```python
from build123d import *

# Parameters (mm, degrees)
RESSALTO_EXTRUS_O1_DEPTH   = 5
ESBO_O2_R                  = 1.35
ESBO_O2_R_2                = 1.373066436
ESBO_O2_R_3                = 1.330065432
ESBO_O2_R_4                = 5
CORTE_EXTRUS_O1_DEPTH      = 137.810087347
ESBO_O3_R                  = 5
CORTE_EXTRUS_O2_DEPTH      = 137.810087347
ESBO_O5_W                  = 31.24115408
ESBO_O5_H                  = 28
CORTE_EXTRUS_O3_DEPTH      = 137.810087347
ESBO_O6_W                  = 5
ESBO_O6_H                  = 28
RESSALTO_EXTRUS_O2_DEPTH   = 2.5
RESSALTO_EXTRUS_O4_DEPTH   = 5
ESBO_O8_R                  = 5
ESBO_O8_R_2                = 1.35
CORTE_EXTRUS_O4_DEPTH      = 135.937948702
ESBO_O10_W                 = 5
ESBO_O10_H                 = 2.5
CORTE_EXTRUS_O5_DEPTH      = 137.985400682
ESBO_O11_W                 = 5
ESBO_O11_H                 = 2.5
RESSALTO_EXTRUS_O5_DEPTH   = 28
ESBO_O14_W                 = 51.545841804
ESBO_O14_H                 = 28
CORTE_EXTRUS_O6_DEPTH      = 10
CORTE_EXTRUS_O7_DEPTH      = 135.822105012
CORTE_EXTRUS_O7_DEPTH_BACK = 10
ESBO_O16_R                 = 5
CORTE_EXTRUS_O8_DEPTH      = 10


with BuildPart() as part:
    # Esboço1 → Ressalto-extrusão1 (new body)
    with BuildSketch(Plane.XY):
        with BuildLine():
            Line((0, -14), (122, -14))
            ThreePointArc((122, -14), (136, 0), (122, 14))
            Line((122, 14), (0, 14))
            ThreePointArc((0, 14), (-14, 0), (0, -14))
        make_face()
    extrude(amount=RESSALTO_EXTRUS_O1_DEPTH)

    # Esboço2 → Corte-extrusão1 (cut, through all)
    with BuildSketch(Plane(origin=(0, 0, 0), x_dir=(-1, 0, 0), z_dir=(0, 0, -1))):
        with Locations((-125.327123404, 10.484762747)):
            Circle(ESBO_O2_R)
        with Locations((-116.938784683, 9.766478358)):
            Circle(ESBO_O2_R)
        with Locations((-111.515237253, 3.327123404)):
            Circle(ESBO_O2_R)
        with Locations((-112.233521642, -5.061215317)):
            Circle(ESBO_O2_R)
        with Locations((-118.672876596, -10.484762747)):
            Circle(ESBO_O2_R_2)
        with Locations((-127.061215317, -9.766478358)):
            Circle(ESBO_O2_R_3)
        with Locations((-132.484762747, -3.327123404)):
            Circle(ESBO_O2_R)
        with Locations((-131.766478358, 5.061215317)):
            Circle(ESBO_O2_R)
        with Locations((-122, 0)):
            Circle(ESBO_O2_R_4)
    extrude(amount=-CORTE_EXTRUS_O1_DEPTH, mode=Mode.SUBTRACT)

    # Esboço3 → Corte-extrusão2 (cut, through all)
    with BuildSketch(Plane(origin=(0, 0, 0), x_dir=(-1, 0, 0), z_dir=(0, 0, -1))):
        Circle(ESBO_O3_R)
    extrude(amount=-CORTE_EXTRUS_O2_DEPTH, mode=Mode.SUBTRACT)

    # Esboço5 → Corte-extrusão3 (cut, through all)
    with BuildSketch(Plane(origin=(0, 0, 0), x_dir=(-1, 0, 0), z_dir=(0, 0, -1))):
        with Locations((-121.62057704, 0)):
            Rectangle(ESBO_O5_W, ESBO_O5_H)
    extrude(amount=-CORTE_EXTRUS_O3_DEPTH, mode=Mode.SUBTRACT)

    # Esboço6 → Ressalto-extrusão2 (add)
    with BuildSketch(Plane(origin=(0, 0, 0), x_dir=(-1, 0, 0), z_dir=(0, 0, -1))):
        with Locations((-103.5, 0)):
            Rectangle(ESBO_O6_W, ESBO_O6_H)
    extrude(amount=RESSALTO_EXTRUS_O2_DEPTH)

    # Esboço7 → Ressalto-extrusão4 (add)
    with BuildSketch(Plane(origin=(0, 0, -2.5), x_dir=(-1, 0, 0), z_dir=(0, 0, -1))):
        with BuildLine():
            Line((-106, 14), (-120, 14))
            ThreePointArc((-120, 14), (-134, 0), (-120, -14))
            Line((-120, -14), (-106, -14))
            Line((-106, -14), (-106, 14))
        make_face()
    extrude(amount=-RESSALTO_EXTRUS_O4_DEPTH)

    # Esboço8 → Corte-extrusão4 (cut, through all)
    with BuildSketch(Plane(origin=(0, 0, -2.5), x_dir=(-1, 0, 0), z_dir=(0, 0, -1))):
        with Locations((-120, 0)):
            Circle(ESBO_O8_R)
        with Locations((-120, 11)):
            Circle(ESBO_O8_R_2)
        with Locations((-109, 0)):
            Circle(ESBO_O8_R_2)
        with Locations((-120, -11)):
            Circle(ESBO_O8_R_2)
        with Locations((-131, 0)):
            Circle(ESBO_O8_R_2)
        with Locations((-112.221825407, 7.778174593)):
            Circle(ESBO_O8_R_2)
        with Locations((-112.221825407, -7.778174593)):
            Circle(ESBO_O8_R_2)
        with Locations((-127.778174593, -7.778174593)):
            Circle(ESBO_O8_R_2)
        with Locations((-127.778174593, 7.778174593)):
            Circle(ESBO_O8_R_2)
    extrude(amount=-CORTE_EXTRUS_O4_DEPTH, mode=Mode.SUBTRACT)

    # Esboço10 → Corte-extrusão5 (cut, through all)
    with BuildSketch(Plane.XZ.offset(14)):
        with Locations((103.5, 3.75)):
            Rectangle(ESBO_O10_W, ESBO_O10_H)
    extrude(amount=-CORTE_EXTRUS_O5_DEPTH, mode=Mode.SUBTRACT)

    # Esboço11 → Ressalto-extrusão5 (add, through all)
    with BuildSketch(Plane.XZ.offset(14)):
        with Locations((98.5, -1.25)):
            Rectangle(ESBO_O11_W, ESBO_O11_H)
    extrude(amount=-RESSALTO_EXTRUS_O5_DEPTH)

    # Esboço14 → Corte-extrusão6 (cut)
    with BuildSketch(Plane(origin=(0, 0, 0), x_dir=(-1, 0, 0), z_dir=(0, 0, -1))):
        with Locations((-10.227079098, 0)):
            Rectangle(ESBO_O14_W, ESBO_O14_H)
    extrude(amount=-CORTE_EXTRUS_O6_DEPTH, mode=Mode.SUBTRACT)

    # Esboço15 → Corte-extrusão7 (cut, two sides: drawn at the far end of the back side and taken through both)
    with BuildSketch(Plane(origin=(0, 0, 0), x_dir=(-1, 0, 0), z_dir=(0, 0, -1)).offset(-CORTE_EXTRUS_O7_DEPTH_BACK)):
        with BuildLine():
            Line((-36, 14), (-50, 14))
            ThreePointArc((-50, 14), (-40.100505063, 9.899494937), (-36, 0))
            Line((-36, 0), (-36, 14))
        make_face()
        with BuildLine():
            Line((-36, -14), (-36, 0))
            ThreePointArc((-36, 0), (-40.100505063, -9.899494937), (-50, -14))
            Line((-50, -14), (-36, -14))
        make_face()
    extrude(amount=CORTE_EXTRUS_O7_DEPTH + CORTE_EXTRUS_O7_DEPTH_BACK, mode=Mode.SUBTRACT)

    # Esboço16 → Corte-extrusão8 (cut)
    with BuildSketch(Plane(origin=(0, 0, 0), x_dir=(-1, 0, 0), z_dir=(0, 0, -1))):
        with Locations((-50, 0)):
            Circle(ESBO_O16_R)
    extrude(amount=-CORTE_EXTRUS_O8_DEPTH, mode=Mode.SUBTRACT)


solid = part.part
```
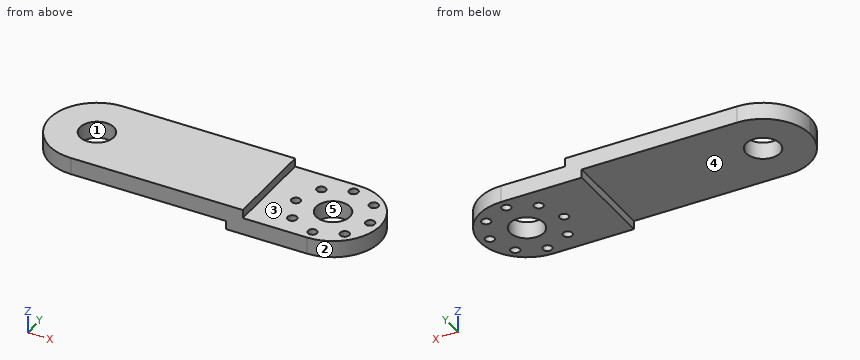
Model file for the job. Use its own axes, mm. Face numbers are marked on the shaded views. A direction names the side the tool comes from. Coordinates: 2 decimals unless noted, no trailing zeros. Loops run counter-clockwise (first coordinate to the right, second up) from the corner with the lowest first, then second, coordinate; pieces in that order, holes last. Notation, with made-up numbers: (69.25, 75.5) - (115.25, 75.5) arc R12 cw to (115.25, 83.5) - close; hole circle Ø7 at (-35, 43). An arc over 180 degrees is marked (long way). Write item = value, one per line. Start each with the question number.
Item 1: Saw through at A-A, the plane x = 109. List the corners of the cut face in (y, z), then the cut area to 4 significant figures.
Item 2: Saw through at C-C, the plane y = 11. List the corners of the cut face in (x, z).
Item 3: Pull direction X, two halves, no side cores. Call the marked faces 1, 2 and 3: +X half, -X half, draft (parallel to the pull), parting line (faces both ways), or undercut.
Item 4: Wall check: probe 1 along X at (y, z) = (7.5, -0.75); probe 2 along Z at (x, y) = (105, 12.5); probe 3 along Z at (x, y) = (69, -3.75). Give the ranges that are in metal, low to high. Write a range as [from, to].
Item 5: 3-axis set-ups, long thin cutter, end or side, ignore diameter. For the marked faces 4 and 5: which of +Z, -Z, +X, -X, +Y, -Y reach the whole face in a straight line?
Item 6: Saw through at D-D, the plane z = 4. List the corners of the cut face in (x, y), then the cut area to 3 significant figures.
Item 7: Saw through at B-B, the plane z = -1.5. State how many separate pieces and enclosed holes the cut face has, then the cut area to 3 significant figures.
Item 8: Drop flat-ended pins along their axis: pin 1 Ø4.5 at (x, y) = (127.78, 7.78) entering from +Z; pin 2 Ø8 at (x, y) = (120, 0) entering from +Z; pin 3 Ø2 at (x, z) = (101.5, 3) entering from +Y; pin 4 Ø4 at (x, y) = (74.5, -10) entering from -Z. Give the stop position or say it passes through.
Answers:
q1.outline = (-14, -2.5) - (-1.35, -2.5) - (-1.35, 2.5) - (-14, 2.5) - close; (1.35, -2.5) - (14, -2.5) - (14, 2.5) - (1.35, 2.5) - close
q1.area = 126.5 mm2
q2.outline = (41.34, 0) - (96, 0) - (96, -2.5) - (118.65, -2.5) - (118.65, 2.5) - (101, 2.5) - (101, 5) - (41.34, 5) - close; (121.35, -2.5) - (128.66, -2.5) - (128.66, 2.5) - (121.35, 2.5) - close
q3.face_1 = undercut
q3.face_2 = +X half
q3.face_3 = draft
q4.probe_1 = [96, 110.9], [113.54, 126.46], [129.1, 131.82]
q4.probe_2 = [-2.5, 2.5]
q4.probe_3 = [0, 5]
q5.face_4 = -Z, -X, +Y, -Y
q5.face_5 = +Z, -Z
q6.outline = (50, -14) - (101, -14) - (101, 14) - (50, 14) arc R14 ccw to start; hole circle Ø10 at (50, 0)
q6.area = 1,660 mm2
q7.separate_pieces = 1
q7.enclosed_holes = 9
q7.area = 856 mm2
q8.pin_1 = 2.5
q8.pin_2 = through
q8.pin_3 = 14
q8.pin_4 = 0
